Answer from the drawing. Dimensions are ordinates in mm from the lowest x, y and z of the part. A direction names the side the tool comes from. Give positions to 0.01 mm unless a question says otherwise; leave off trailing zeros.
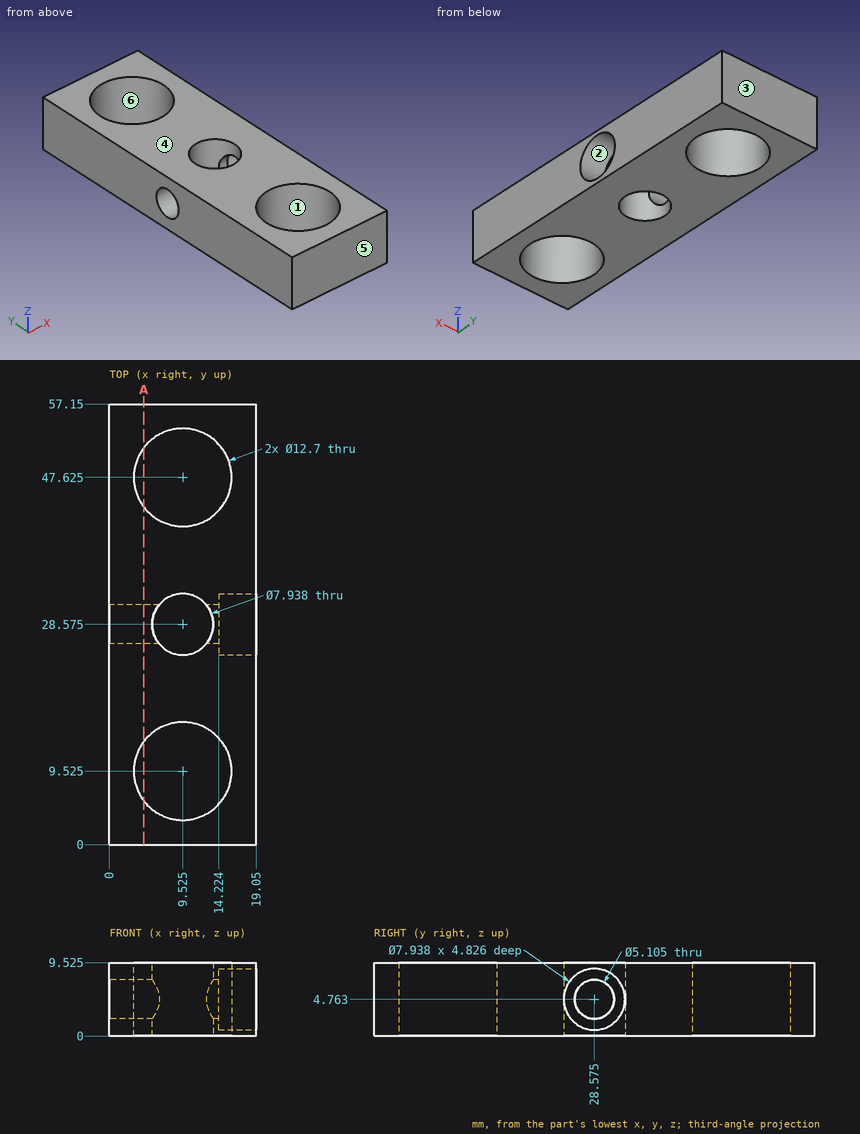
1. The mould has two halves that part along Y. Classify the marked faces 3, 4, 5 and 6: pulls with the +Y half, pulls with the -Y half, needs draft (parallel to the pull), parting line crosses it, or undercut.
Findings below:
face 3: pulls with the +Y half
face 4: needs draft
face 5: pulls with the -Y half
face 6: undercut
2. The part is cut by section A-A (x = 4.5). State how many separate pieces and enclosed holes the cut face has, then the cut area to 3 significant figures.
Findings below:
separate pieces: 3
enclosed holes: 1
area: 376 mm2
3. Which of the six approach directions +Z, -Z, +X, -X, +Y, -Y give full straight-line access (tool end or side, diameter ignored) to the marked faces 1 and 2?
Findings below:
face 1: +Z, -Z
face 2: +X
4. Straight lines are drawn through the part: probe 1 along Y at (x, z) = (14.5, 4.25); probe 2 along X at (y, z) = (11, 9); probe 3 along X at (y, z) = (10.5, 3). For each, find the intervals that lie inside material, in ascending order.
Findings below:
probe 1: y = 0 to 5.58, 13.47 to 24.64, 32.51 to 43.68, 51.57 to 57.15
probe 2: x = 0 to 3.35, 15.7 to 19.05
probe 3: x = 0 to 3.25, 15.8 to 19.05
